Autodesk Inventor part; units mm, degrees
ref_plane "YZ Plane" through (0, 0, 0) normal (1, 0, 0) x (0, 1, 0)
ref_plane "XZ Plane" through (0, 0, 0) normal (0, 1, 0) x (-1, 0, 0)
ref_plane "XY Plane" through (0, 0, 0) normal (0, 0, 1) x (1, 0, 0)
sketch "Sketch1" plane through (0, 0, 0) normal (1, 0, 0) x (0, 1, 0)
  line L0 (0, 0) -> (0, -4.6)
  line L1 (0, -4.6) -> (20, -4.6)
  line L2 (20, -4.6) -> (20, -1)
  line L3 (20, -1) -> (6, -1)
  line L4 (6, -1) -> (5, 0)
  line L5 (5, 0) -> (0, 0)
  dimension "d1" = 20
  dimension "d2" = 5
  dimension "d3" = 3.6
  dimension "d4" = 4.6
  dimension "d5" = 1
extrude "Extrusion1" add sketch "Sketch1" along normal blind 30
chamfer "Chamfer1" distance 2 angle 45 1 edges at (0, 20, -2.8)
sketch "Sketch2" plane through (0, 6, -1) normal (0, 0, 1) x (1, 0, 0)
  circle A0 centre (15, 5) radius 1.6
  line L0 (0, -6) -> (30, -6)
  line L1 (30, 14) -> (30, 0)
  dimension "d11" = 11
  dimension "d12" = 3.2
  dimension "d13" = 15
hole "Hole1" at (15, 11, -1) direction (0, 0, -1) diameter 3 depth 10 tip angle 118
properties part number "BrueckenGR_LVE2560E"
The listing builds one solid part. Answer for the finished solid, in the listing's coordinates (mm). A direction names the side the tool comes from. Coordinates: 2 decimals unless noted, no trailing zeros. Order: outer loops, then holes, each group sorted by start corner. A loop starts at its lowest first (then second) coordinate and runs counter-clockwise, first axis right, second up. Notation, with made-up numbers: (43.5, 11) -> (75.5, 11) arc R34 cw to (75.5, 47) -> close; hole circle Ø3 at (48.5, -6). An arc over 180 degrees is marked (long way). Answer in a Markdown table with one row per item. Add a question column.
Item 1: Find section D-D (x = 24.5). Write down the section's boundary in (y, z), then the cut area to 3 significant figures.
Item 2: Find section A-A (y = 11). Write down the section's boundary in (x, z), then the cut area to 3 significant figures.
Item 3: Find section B-B (z = -4.15). Write down the section's boundary in (x, y), then the cut area to 3 significant figures.
Item 4: Find section C-C (x = 15). Write down the section's boundary in (y, z), then the cut area to 3 significant figures.
Item 5: Determine the mould class of faces 3 (the face through (14.93, 12.5, -2.83)), 4 (the face through (0, 9, -3)), 5 (the face through (16, 20, -3)) for opening direction X: +X half, -X half, draft (parallel to the pull), parting line (faces both ways), or undercut.
Item 6: Each of these flat-tipped pins is pushed along its axis until it touches: P1, Ø1.8, axis at x = 15, y = 11, coming from the -Z side; P2, Ø7, axis at x = 8, y = 11.5, coming from the +Z side. Where does it stop, or does it pass through?
Item 7: Which of the six approach directions +Z, -Z, +X, -X, +Y, -Y give full straight-line access (tool end or side, diameter ignored) to faces 1 (the face through (15, 3, 0)), 2 (the face through (15, 13, -1))?
Item 8: Find the intervals of material crossed by L1, parallel to Y at x = 15, z = -3.5; L2, parallel to X at y = 11, z = -1.95; L3, parallel to Z at x = 19, y = 16.25, in increasing order. Write a range as from..to.
Result set:
| question | item | result |
|---|---|---|
| 1 | outline | (0, -4.6) -> (20, -4.6) -> (20, -1) -> (6, -1) -> (5, 0) -> (0, 0) -> close |
| 1 | area | 77.5 mm² |
| 2 | outline | (0, -4.6) -> (13.5, -4.6) -> (13.5, -1) -> (0, -1) -> close; (16.5, -4.6) -> (30, -4.6) -> (30, -1) -> (16.5, -1) -> close |
| 2 | area | 97.2 mm² |
| 3 | outline | (0, 0) -> (30, 0) -> (30, 20) -> (2, 20) -> (0, 18) -> close; hole circle Ø3 at (15, 11) |
| 3 | area | 591 mm² |
| 4 | outline | (0, -4.6) -> (9.5, -4.6) -> (9.5, -1) -> (6, -1) -> (5, 0) -> (0, 0) -> close; (12.5, -4.6) -> (20, -4.6) -> (20, -1) -> (12.5, -1) -> close |
| 4 | area | 66.7 mm² |
| 5 | face 3 | undercut |
| 5 | face 4 | -X half |
| 5 | face 5 | draft |
| 6 | P1 | passes through |
| 6 | P2 | stops at z = -1 |
| 7 | face 1 | +Z, +X, -X, +Y, -Y |
| 7 | face 2 | +Z, +X, -X, +Y |
| 8 | L1 | y = 0..9.5, 12.5..20 |
| 8 | L2 | x = 0..13.5, 16.5..30 |
| 8 | L3 | z = -4.6..-1 |
